Input: part model. Units: mm. Frame: model coordinates. A direction names the side the tool comes from. Give positions to 0.01 mm unless a question says otherwise; leave off trailing zeros. Order: outer loops, then holes, each group sorted by start corner. A loop starts at its lowest first (then second) coordinate and runs counter-clockwise, first axis right, second up. Notation, with made-up numbers: (35.5, 23.25) -> (77.5, 23.25) arc R7 cw to (77.5, 30.25) -> close; hole circle Ø7 at (55.5, 51.5). An arc over 180 degrees is marked (long way). Use a Markdown table: item, result. Add a question column.
from build123d import *

# Parameters (mm, degrees)
ESQUISSE1_W        = 87
ESQUISSE1_H        = 75
BOSS_EXTRU_1_DEPTH = 1
ESQUISSE2_W        = 10
ESQUISSE2_H        = 20
BOSS_EXTRU_2_DEPTH = 5


with BuildPart() as part:
    # Esquisse1 → Boss.-Extru.1 (new body)
    with BuildSketch(Plane.XY):
        with Locations((10.327168808, -6.216535433)):
            Rectangle(ESQUISSE1_W, ESQUISSE1_H)
    extrude(amount=BOSS_EXTRU_1_DEPTH)

    # Esquisse2 → Boss.-Extru.2 (add)
    with BuildSketch(Plane.ZY.offset(33.172831192)):
        with Locations((-4, -6.216535433)):
            Rectangle(ESQUISSE2_W, ESQUISSE2_H)
    extrude(amount=-BOSS_EXTRU_2_DEPTH)


solid = part.part
Q1. First-contact query: pin 1 (4 mm diameter, centred on x = -31.5, z = -5, fed in from +Y); pin 2 (4 mm diameter, centred on x = -29.5, z = -3, fed in from -Y); pin 3 (1 mm diameter, centred on y = -30.5, z = -1, fed in from +X); pin 4 (6 mm diameter, centred on x = -4.5, y = -19, fed in from -Z). Flat tips, straight axial feed; report the tip coordinate or a pass-through.
Q2. Access query for faces 1 (the flat face through (-31, -16.217, -5)), 2 (the flat face through (-28.173, -6, -5)), 3 (the flat face through (-31, 3.783, -5)). Directions: +Z, -Z, +X, -X, +Y, -Y. A direction counts if a zero-diameter tool reaches every point of the face in a straight line with its end or side. Return the directions, or none.
Q3. Section query B-B (y = 23). Return loops of the section in (x, z).
Q4. Section query A-A (x = -9). Return loops of the section in (y, z), plus the area to 3 significant figures.
Q5. Ray query, line 1 (X direction, y = -14.5, z = -2.5); line 2 (Z direction, x = 4, y = -24.5). Return the intervals inside material, ascending.
Solution:
| question | item | result |
|---|---|---|
| 1 | pin 1 | stops at y = 3.78 |
| 1 | pin 2 | stops at y = -16.22 |
| 1 | pin 3 | passes through |
| 1 | pin 4 | stops at z = 0 |
| 2 | face 1 | -Z, +X, -X, -Y |
| 2 | face 2 | -Z, +X, +Y, -Y |
| 2 | face 3 | -Z, +X, -X, +Y |
| 3 | outline | (-33.17, 0) -> (53.83, 0) -> (53.83, 1) -> (-33.17, 1) -> close |
| 4 | outline | (-43.72, 0) -> (31.28, 0) -> (31.28, 1) -> (-43.72, 1) -> close |
| 4 | area | 75.0 mm² |
| 5 | line 1 | x = -33.17 to -28.17 |
| 5 | line 2 | z = 0 to 1 |
